from build123d import *

# Parameters (mm, degrees)
F0_W     = 42
F0_H     = 32
F1_DEPTH = 11
F2_W     = 10
F2_H     = 11
F3_DEPTH = 25.4
F4_DEPTH = 25.4
F7_DEPTH = 1.525342


with BuildPart() as f1:
    # F0 (on Front) → F1 (new body)
    with BuildSketch(Plane.XZ):
        with Locations((-6.920929, -1.405328)):
            Rectangle(F0_W, F0_H)
    extrude(amount=F1_DEPTH)

    # F2 (on face) → F3 (cut)
    with BuildSketch(Plane.XY.offset(14.594672)):
        with Locations((-22.920929, -5.5)):
            Rectangle(F2_W, F2_H)
    extrude(amount=-F3_DEPTH, mode=Mode.SUBTRACT)

    # F2 (on face) → F4 (cut)
    with BuildSketch(Plane.XY.offset(14.594672)):
        with Locations((9.079071, -5.5)):
            Rectangle(F2_W, F2_H)
    extrude(amount=-F4_DEPTH, mode=Mode.SUBTRACT)

    # F6 (on face) → F7 (join)
    with BuildSketch(Plane(origin=(0, 0, 0), x_dir=(-1, 0, 0), z_dir=(0, 1, 0))):
        with BuildLine():
            ThreePointArc((14.309347, 11.993863), (13.754616, 12.312149), (13.150224, 12.521295))
            ThreePointArc((13.150224, 12.521295), (12.905231, 11.705894), (13.101386, 10.877388))
            ThreePointArc((13.101386, 10.877388), (13.439924, 11.24292), (13.917749, 11.384008))
            ThreePointArc((13.917749, 11.384008), (14.074362, 11.714097), (14.309347, 11.993863))
        make_face()
    extrude(amount=-F7_DEPTH)


solid = f1.part
Can you work these out from the model? Positions are in its coordinate system, mm. A direction names the side the tool comes from. Round coordinates to 2 decimals unless told otherwise and drop trailing zeros. Write each loop counter-clockwise with the first axis right and the second up, starting at its lowest first coordinate (ties: lowest second). Pieces come first, ordered by that corner, then holes. Notation, with made-up numbers: M 25,82.5 L 40,82.5 A22 ccw 40,110.5 Z; hole C 36,43 d2. An arc over 180 degrees is marked long. Use a Markdown table: item, result.
Item 1: Which directions (+Z, -Z, +X, -X, +Y, -Y) give clear straight access to the entire face, cutting with the end or side of a thin tool? Please do faces 1 (the face through (-23, -5, -10.805)), 2 (the face through (9, -5, -10.805)), 3 (the face through (14.079, -5, -14)).
Found:
| item | result |
|---|---|
| face 1 | +Z, -X, +Y, -Y |
| face 2 | +Z, +X, +Y, -Y |
| face 3 | +Z, -Z, +X, +Y, -Y |
Item 2: I want a section at C-C (z = -8.5). List the corners of the cut face in (x, y) for me.
Found:
| item | result |
|---|---|
| outline | M -17.92,-11 L 4.08,-11 L 4.08,0 L -17.92,0 Z |
Item 3: I want a section at B-B (x = -22.5). List the corners of the cut face in (y, z) for me, and give its area (3 significant figures).
Found:
| item | result |
|---|---|
| outline | M -11,-17.41 L 0,-17.41 L 0,-10.81 L -11,-10.81 Z |
| area | 72.6 mm2 |
Item 4: If I drill on line 1 along X through (y, z) = (-2, 3); line 2 along Z through (x, y) = (11.5, -3.25), over which ranges is the centre line in solid material (lowest first)? Write a range as [from, to].
Found:
| item | result |
|---|---|
| line 1 | x = [-17.92, 4.08] |
| line 2 | z = [-17.41, -10.81] |
Item 5: I want a section at A-A (y = -8.75). List the corners of the cut face in (x, z) for me.
Found:
| item | result |
|---|---|
| outline | M -27.92,-17.41 L 14.08,-17.41 L 14.08,-10.81 L 4.08,-10.81 L 4.08,14.59 L -17.92,14.59 L -17.92,-10.81 L -27.92,-10.81 Z |
Item 6: For pin 1 Ø5 at (x, y) = (-22.5, -4) entering from +Z; pin 2 Ø1 at (y, z) = (-3, 8.5) entering from -X, each with a flat end and sliding along its axis, tell me the tip position at first contact or that it passes through.
Found:
| item | result |
|---|---|
| pin 1 | stops at z = -10.81 |
| pin 2 | stops at x = -17.92 |
